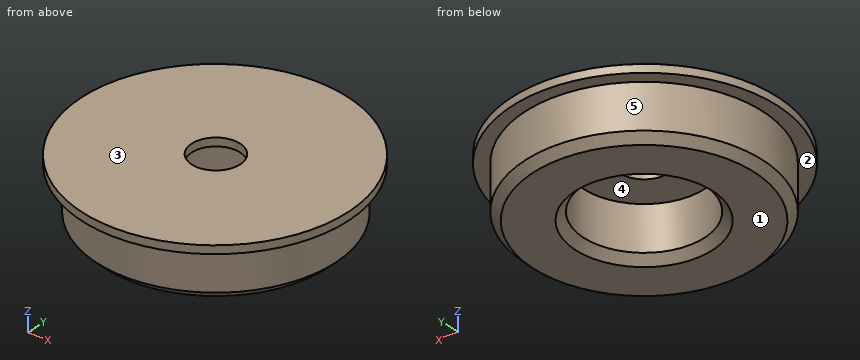
```python
from build123d import *

# Parameters (mm, degrees)
F0_R     = 16.5
F1_DEPTH = 1
F2_R     = 14.75
F3_DEPTH = 6.5
F4_R     = 3
F5_DEPTH = 25
F6_R     = 7.5
F7_DEPTH = 6.5
F8_SIZE  = 1


with BuildPart() as f1:
    # F0 (on Top) → F1 (new body)
    with BuildSketch(Plane.XY):
        with Locations((1e-06, -0.140358)):
            Circle(F0_R)
    extrude(amount=F1_DEPTH)

    # F2 (on face) → F3 (join)
    with BuildSketch(Plane(origin=(0, 0, 0), x_dir=(1, 0, 0), z_dir=(0, 0, -1))):
        Circle(F2_R)
    extrude(amount=F3_DEPTH)

    # F4 (on face) → F5 (cut)
    with BuildSketch(Plane(origin=(0, 0, -6.5), x_dir=(1, 0, 0), z_dir=(0, 0, -1))):
        Circle(F4_R)
    extrude(amount=-F5_DEPTH, mode=Mode.SUBTRACT)

    # F6 (on face) → F7 (cut, through all)
    with BuildSketch(Plane(origin=(0, 0, -6.5), x_dir=(1, 0, 0), z_dir=(0, 0, -1))):
        Circle(F6_R)
    extrude(amount=-F7_DEPTH, mode=Mode.SUBTRACT)

    # F8
    f8_edges = [f1.edges().sort_by_distance(p)[0] for p in [
        (-7.5, 0, -6.5),
        (-14.75, 0, -6.5),
    ]]
    chamfer(f8_edges, length=F8_SIZE)


solid = f1.part
```
The listing builds one solid part. Answer for the finished solid, in the listing's coordinates (mm). Face numbers are marked on the shaded views. A direction names the side the tool comes from. Round coordinates to 2 decimals unless told otherwise and drop trailing zeros. Loops run counter-clockwise (first coordinate to the right, second up) from the corner with the lowest first, then second, coordinate; pieces in that order, holes last. Notation, with made-up numbers: (9, 47) - (13, 47) arc R25 ccw to (13, 60) - close; hole circle Ø8 at (77.5, -38). An arc over 180 degrees is marked (long way). Use one line per item in the form item = value. Start each with the question number.
1. A tool of negligible diameter and unlimited length cuts with its end or side. For the marked faces 1 and 2, from which of +Z, -Z, +X, -X, +Y, -Y can it reach the whole face along a straight path? Write none if from no direction.
2. Given pin 1 Ø4 at (y, z) = (12, -2.5) entering from -X; pin 2 Ø4 at (y, z) = (3.5, -3.5) entering from +X; pin 3 Ø5.5 at (x, y) = (0, 0) entering from -Z; pin 4 Ø3 at (y, z) = (-13, -0.5) entering from +X, each flat-ended and moving along its own axis, determine where each tip first touches the part or whether it passes through.
3. For a pull along X with two mould halves and no side action, classify the marked faces 3, 4 and 5 as pulls with the +X half, pulls with the -X half, needs draft (parallel to the pull), parting line crosses it, or undercut.
4. Consider line 1 (X direction, y = 0, z = 0.3); line 2 (X direction, y = 0, z = -3.6). Determine where each line is inside the solid, lowest interval first. Write a range as [from, to].
5. The part is cut by section B-B on z = -2.5. Determine the outline of the cut face in (x, y), then the cut area to 3 significant figures.
6. The part is cut by section A-A on x = 0. Determine the outline of the cut face in (y, z), then the cut area to 3 significant figures.
Geometry check:
q1.face_1 = -Z, +X, -X, +Y, -Y
q1.face_2 = -Z
q2.pin_1 = -10.84
q2.pin_2 = 14.67
q2.pin_3 = through
q2.pin_4 = 11.88
q3.face_3 = needs draft
q3.face_4 = undercut
q3.face_5 = parting line crosses it
q4.line_1 = [-16.5, -3], [3, 16.5]
q4.line_2 = [-14.75, -7.5], [7.5, 14.75]
q5.outline = circle Ø29.5 at (0, 0); hole circle Ø15 at (0, 0)
q5.area = 507 mm^2
q6.outline = (-16.64, 0) - (-14.75, 0) - (-14.75, -5.5) - (-13.75, -6.5) - (-8.5, -6.5) - (-7.5, -5.5) - (-7.5, 0) - (-3, 0) - (-3, 1) - (-16.64, 1) - close; (3, 0) - (7.5, 0) - (7.5, -5.5) - (8.5, -6.5) - (13.75, -6.5) - (14.75, -5.5) - (14.75, 0) - (16.36, 0) - (16.36, 1) - (3, 1) - close
q6.area = 119 mm^2
